Autodesk Inventor part; units mm, degrees
ref_plane "YZ Plane" through (0, 0, 0) normal (1, 0, 0) x (0, 1, 0)
ref_plane "XZ Plane" through (0, 0, 0) normal (0, 1, 0) x (-1, 0, 0)
ref_plane "XY Plane" through (0, 0, 0) normal (0, 0, 1) x (1, 0, 0)
sketch "Sketch1" plane through (0, 0, 0) normal (0, 0, 1) x (1, 0, 0)
  line L0 (0, 0) -> (25.4, 0)
  line L1 (25.4, 0) -> (25.4, 25.4)
  line L2 (25.4, 25.4) -> (0, 25.4)
  line L3 (0, 25.4) -> (0, 0)
  line L4 (3.175, 22.225) -> (22.225, 22.225)
  line L5 (22.225, 22.225) -> (22.225, 3.175)
  line L6 (22.225, 3.175) -> (3.175, 3.175)
  line L7 (3.175, 3.175) -> (3.175, 22.225)
  dimension "d0" = 25.4
  dimension "d1" = 25.4
  dimension "d2" = 3.175
extrude "Extrusion1" add sketch "Sketch1" against normal blind 590.55
sketch "Sketch4" plane through (0, 25.4, 0) normal (0, 1, 0) x (1, 0, 0)
  line L0 (25.4, 590.55) -> (0, 590.55)
  line L1 (25.4, 0) -> (0, 0)
  point P0 (12.7, 12.7)
  point P1 (12.7, 38.1)
  point P2 (12.7, 577.85)
  point P3 (12.7, 552.45)
  point P4 (12.7, 527.05)
  dimension "d32" = 12.7
  dimension "d33" = 25.4
  dimension "d34" = 12.7
  dimension "d35" = 25.4
  dimension "d36" = 25.4
hole "Hole4" at (12.7, 25.4, -12.7) at (12.7, 25.4, -38.1) at (12.7, 25.4, -577.85) at (12.7, 25.4, -552.45) at (12.7, 25.4, -527.05) direction (0, -1, 0) diameter 5.08 depth 25.4 tip angle 118
properties part number "new horizontall kicker thing"
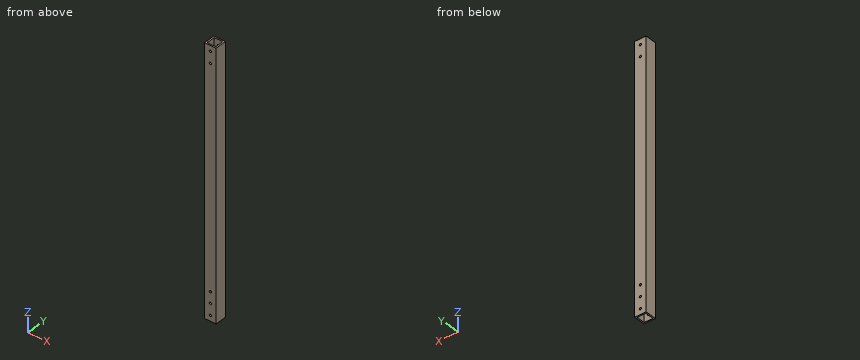
Model file for the job. Use its own axes, mm. Round coordinates to 2 decimals unless told otherwise and drop trailing zeros. Order: outer loops, then holes, each group sorted by start corner. A loop starts at its lowest first (then second) coordinate and runs counter-clockwise, first axis right, second up.
(1) Drill centre lines: line 1 (Z direction, x = 12.7, y = 1.25); line 2 (X direction, y = 16.5, z = -413) (3 decimals); line 3 (X direction, y = 2.3, z = -38.1). Where is each one in solid material? Low to high.
(2) Band-saw the part on B-B (z = -111). List the corners of the cut face in (x, y) (3 decimals).
(3) Band-saw the part on A-A (y = 14.25). List the corners of the cut face in (x, z) (3 decimals).
(4) Pin check, flat tip, straight feed: pin 1 (4.5 mm diameter, centred on x = 12.7, z = -552.45, fed in from +Y). Stop position of the tip, or through.
Verdict:
1. line 1: z = -590.55 to -580.39, -575.31 to -554.99, -549.91 to -529.59, -524.51 to -40.64, -35.56 to -15.24, -10.16 to 0
1. line 2: x = 0 to 3.175, 22.225 to 25.4
1. line 3: x = 0 to 10.16, 15.24 to 25.4
2. outline: (0, 0) - (25.4, 0) - (25.4, 25.4) - (0, 25.4) - close; hole (3.175, 3.175) - (22.225, 3.175) - (22.225, 22.225) - (3.175, 22.225) - close
3. outline: (0, -590.55) - (3.175, -590.55) - (3.175, 0) - (0, 0) - close; (22.225, -590.55) - (25.4, -590.55) - (25.4, 0) - (22.225, 0) - close
4. pin 1: passes through
